```python
from build123d import *

# Parameters (mm, degrees)
CYLINDER007_R     = 0.5
CYLINDER007_DEPTH = 2.51
CYLINDER008_R     = 0.9
CYLINDER008_DEPTH = 5.05


with BuildPart() as cylinder007:
    # Cylinder007 → Cylinder007 (new body)
    with BuildSketch(Plane(origin=(2.54, 0, -2.51), x_dir=(1, 0, 0), z_dir=(0, 0, 1))):
        Circle(CYLINDER007_R)
    extrude(amount=CYLINDER007_DEPTH)


with BuildPart() as cone003:
    # Cone003 → Cone003 (revolve)
    with BuildSketch(Plane(origin=(2.54, 0, -3.51), x_dir=(1, 0, 0), z_dir=(0, -1, 0))):
        Polygon((0, 0), (0.1, 0), (0.5, 1), (0, 1), align=None)
    revolve(axis=Axis((2.54, 0, -3.51), (0, 0, 1)))


with BuildPart() as fusion003:
    # Cylinder008 → Cylinder008 (new body)
    with BuildSketch(Plane(origin=(2.54, 0, 0), x_dir=(1, 0, 0), z_dir=(0, 0, 1))):
        Circle(CYLINDER008_R)
    extrude(amount=CYLINDER008_DEPTH)

    # Fusion003: union Cylinder007, Cone003
    add(cylinder007.part)
    add(cone003.part)


with BuildPart() as fusion003_1:
    # Fusion003 placement: moved
    add(fusion003.part.moved(Location((45.72, 13.97, 0))))


solid = fusion003_1.part
```
Work out the finished part from the listing and answer in its coordinate system (mm). A direction names the side the tool comes from. Give positions to 0.01 mm unless a question says otherwise; leave off trailing zeros. Loops run counter-clockwise (first coordinate to the right, second up) from the corner with the lowest first, then second, coordinate; pieces in that order, holes last. Notation, with made-up numbers: (81.25, 28) - (136.25, 28) arc R21 cw to (136.25, 36) - close; hole circle Ø8 at (80.25, -32.5). An arc over 180 degrees is marked (long way). Use CSV: the item, a comma, the result in double quotes. Start each with the question number.
(1) Find section C-C, the plane z = 3.5. Determine the outline of the cut face in (x, y).
(2) Find the intervals of material crossed by L1, parallel to Z at x = 48.9, y = 14.2; L2, parallel to Z at x = 48.7, y = 14.1; L3, parallel to X at y = 14.15, z = -2.5, in increasing order.
(3) Find section D-D, the plane y = 13.3. Determine the outline of the cut face in (x, z).
(4) A tool of negligible diameter and unlimited length cuts with its end or side. For faces 1 (the face through (49, 14, 0)), 2 (the face through (48, 14, 5.05)), from which of +Z, -Z, +X, -X, +Y, -Y can it reach the whole face along a straight path? Write none if from no direction.
(5) Find section B-B, the plane x = 48.26. Determine the outline of the cut face in (y, z), plus the area to 3 significant figures.
(6) Find section A-A, the plane y = 13.97. Determine the outline of the cut face in (x, z).
Results found:
1,outline,"circle Ø1.8 at (48.26, 13.97)"
2,L1,"0 to 5.05"
2,L2,"-2.61 to 5.05"
2,L3,"47.79 to 48.73"
3,outline,"(47.66, 0) - (48.86, 0) - (48.86, 5.05) - (47.66, 5.05) - close"
4,face 1,"-Z"
4,face 2,"+Z, +X, -X, +Y, -Y"
5,outline,"(13.07, 0) - (13.47, 0) - (13.47, -2.51) - (13.87, -3.51) - (14.07, -3.51) - (14.47, -2.51) - (14.47, 0) - (14.87, 0) - (14.87, 5.05) - (13.07, 5.05) - close"
5,area,"12.2 mm^2"
6,outline,"(47.36, 0) - (47.76, 0) - (47.76, -2.51) - (48.16, -3.51) - (48.36, -3.51) - (48.76, -2.51) - (48.76, 0) - (49.16, 0) - (49.16, 5.05) - (47.36, 5.05) - close"
